Autodesk Inventor part; units mm, degrees
ref_plane "YZ Plane" through (0, 0, 0) normal (1, 0, 0) x (0, 1, 0)
ref_plane "XZ Plane" through (0, 0, 0) normal (0, 1, 0) x (-1, 0, 0)
ref_plane "XY Plane" through (0, 0, 0) normal (0, 0, 1) x (1, 0, 0)
sketch "Sketch1" plane through (0, 0, 0) normal (1, 0, 0) x (0, 1, 0)
  line L0 (22.5, 15.5) -> (0, 15.5)
  line L1 (0, 15.5) -> (0, -15.5)
  line L2 (0, -15.5) -> (22.5, -15.5)
  line L3 (22.5, -15.5) -> (22.5, 15.5)
  line L4 (0, -21.7) -> (0, 21.7)
  point P0 (0, 0)
  point P1 (22.5, 0)
  dimension "d0" = 31
  dimension "d1" = 22.5
extrude "Extrusion1" add sketch "Sketch1" along normal mid plane 3.5
sketch "Sketch2" plane through (1.75, 0, 0) normal (1, 0, 0) x (0, 0, -1)
  line L0 (-10.2455, 0) -> (0, 17.076)
  line L1 (0, 17.076) -> (10.2455, 0)
  line L2 (-15.5, 0) -> (15.5, 0)
  point P0 (0, 0)
  dimension "d31" = 20.491
  dimension "d33" = 17.076
extrude "Extrusion4" add sketch "Sketch2" along normal blind 2.5
mirror "Mirror2" about plane through (0, 0, 0) normal (1, 0, 0) of "Extrusion4"
sketch "Sketch7" plane through (-1.75, 0, -15.5) normal (0, -1, 0) x (1, 0, 0)
  line L0 (0, 0) -> (3.5, 0)
  line L1 (3.5, 5.2545) -> (3.5, 0)
  line L2 (3.5, 5.2545) -> (6, 5.2545)
  line L3 (6, 25.7455) -> (6, 5.2545)
  line L4 (3.5, 25.7455) -> (6, 25.7455)
  line L5 (3.5, 31) -> (3.5, 25.7455)
  line L6 (0, 31) -> (3.5, 31)
  line L7 (0, 25.7455) -> (0, 31)
  line L8 (0, 25.7455) -> (-2.5, 25.7455)
  line L9 (-2.5, 25.7455) -> (-2.5, 5.2545)
  line L10 (0, 5.2545) -> (-2.5, 5.2545)
  line L11 (0, 0) -> (0, 5.2545)
  point P0 (1.75, 15.5)
extrude "Extrusion5" add sketch "Sketch7" along normal blind 12
sketch "Sketch8" plane through (4.25, 0, -10.2455) normal (0, 0, -1) x (-1, 0, 0)
  line L0 (2.5, 0) -> (0, 0)
  line L1 (0, 0) -> (0, -12)
  line L2 (2.5, -12) -> (0, -12)
  line L3 (2.5, 0) -> (2.5, -12)
  point P0 (4.25, 0)
extrude "Extrusion6" add sketch "Sketch8" along normal up to surface (5.2545 mm away)
mirror "Mirror3" about plane through (0, 0, 0) normal (0, 0, 1) of "Extrusion6"
mirror "Mirror4" about plane through (0, 0, 0) normal (1, 0, 0) of "Extrusion6", "Mirror3"
sketch "Sketch9" plane through (4.25, 0, 0) normal (1, 0, 0) x (0, 0, -1)
  line L0 (0, 17.076) -> (-10.2455, 0) construction
  line L1 (0, 17.076) -> (0, -12) construction
  line L2 (-15.5, -12) -> (15.5, -12) construction
  line L3 (-5.1228, 8.538) -> (5.1227, 8.538) construction
  line L4 (0, 17.076) -> (10.2455, 0) construction
  line L5 (-7.5227, 4.538) -> (7.5227, 4.538) construction
  line L6 (-13.5227, -5.462) -> (13.5227, -5.462) construction
  point P0 (0, 0)
  dimension "d40" = 4
  dimension "d50" = 10
hole "Hole3" at (4.25, 4.538, 0) direction (-1, 0, 0) diameter 4.5 end through all countersink diameter 9 countersink angle 90
hole "Hole4" at (4.25, -5.462, 0) direction (-1, 0, 0) diameter 4.5 end through all countersink diameter 9 countersink angle 90
chamfer "Chamfer1" distance 8 angle 45 2 edges at (0, 22.5, 15.5) (0, 22.5, -15.5)
properties part number "Traingular Hopper Connector"
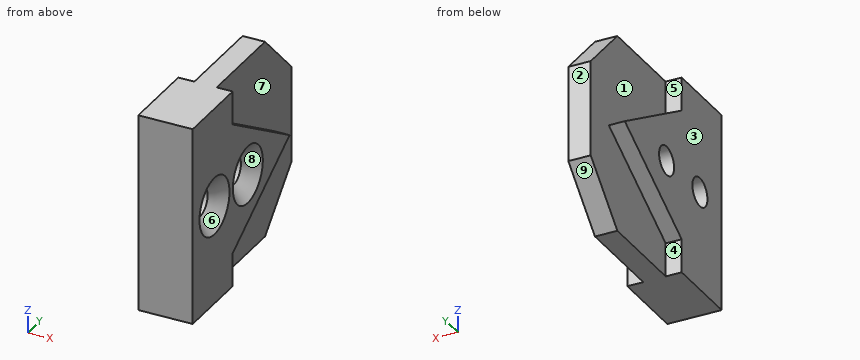
Read the model definition and answer for the solid it produces. Units are mm, in the model's axes. Face numbers are marked on the shaded views. A direction names the side the tool comes from. Coordinates: 2 decimals unless noted, no trailing zeros. Write each loop counter-clockwise with the first axis right and the second up, starting at its lowest first coordinate (ties: lowest second). Pieces come first, ordered by that corner, then holes. Notation, with made-up numbers: (85, -23.75) -> (135, -23.75) arc R34 cw to (135, 8.25) -> close; hole circle Ø5 at (37, 21.25). An arc over 180 degrees is marked (long way). Answer as a JSON object with one key per item and string values.
Q1. Determine the mould class of the marked faces 6, 7, 8 and 9 for opening direction Z: pulls with the +Z half, pulls with the -Z half, needs draft (parallel to the pull), parting line crosses it, or undercut.
The answers:
{"face 6": "undercut", "face 7": "needs draft", "face 8": "undercut", "face 9": "pulls with the -Z half"}
Q2. The part is cut by section C-C on y = 18.5. Give the vertices of the cut face in (x, z).
The answers:
{"outline": "(-1.75, -11.5) -> (1.75, -11.5) -> (1.75, 11.5) -> (-1.75, 11.5) -> close"}
Q3. Consider line 1 (Y direction, x = 0.5, z = 0); line 2 (Y direction, x = 0.75, z = -0.5); line 3 (X direction, y = 17.5, z = -2). Determine where each line is inside the solid, lowest interval first. Write a range as [from, to].
The answers:
{"line 1": "y = [-12, -7.71], [-3.21, 2.29], [6.79, 22.5]", "line 2": "y = [-12, -7.66], [-3.27, 2.34], [6.73, 22.5]", "line 3": "x = [-1.75, 1.75]"}
Q4. The part is cut by section A-A on x = -3. Give the vertices of the cut face in (y, z), then the cut area to 3 significant figures.
The answers:
{"outline": "(-12, -15.5) -> (0, -15.5) -> (0, -10.25) -> (17.08, 0) -> (0, 10.25) -> (0, 15.5) -> (-12, 15.5) -> close; hole circle Ø4.5 at (-5.46, 0); hole circle Ø4.5 at (4.54, 0)", "area": "515 mm2"}
Q5. Flat-ended cylindrical pins translate along their axes: pin 1 Ø7 at (y, z) = (-5.462, 0) entering from -X; pin 2 Ø2 at (x, z) = (3.5, 14) entering from +Y; pin 3 Ø2 at (y, z) = (7.5, -10.5) entering from -X; pin 4 Ø2 at (y, z) = (17.5, -8) entering from +X. Find the tip coordinate at first contact, or state that the pin passes through.
The answers:
{"pin 1": "stops at x = -4.25", "pin 2": "stops at y = 0", "pin 3": "stops at x = -1.75", "pin 4": "stops at x = 1.75"}
Q6. The part is cut by section B-B on z = -12.5. Give the vertices of the cut face in (x, y), then the cut area to 3 significant figures.
The answers:
{"outline": "(-4.25, -12) -> (4.25, -12) -> (4.25, 0) -> (1.75, 0) -> (1.75, 17.5) -> (-1.75, 17.5) -> (-1.75, 0) -> (-4.25, 0) -> close", "area": "163 mm2"}
Q7. The part is cut by section D-D on z = 11. Give the vertices of the cut face in (x, y), then the cut area to 4 significant figures.
The answers:
{"outline": "(-4.25, -12) -> (4.25, -12) -> (4.25, 0) -> (1.75, 0) -> (1.75, 19) -> (-1.75, 19) -> (-1.75, 0) -> (-4.25, 0) -> close", "area": "168.5 mm2"}
Q8. A tool of negligible diameter and unlimited length cuts with its end or side. For the marked faces 1, 2, 3, 4 and 5, from which of +Z, -Z, +X, -X, +Y, -Y can it reach the whole face along a straight path? Write none if from no direction.
The answers:
{"face 1": "-X, +Y", "face 2": "+Z, -Z, +X, -X, +Y", "face 3": "+Z, -Z, -X, +Y, -Y", "face 4": "-Z, -X, +Y", "face 5": "+Z, -X, +Y"}
